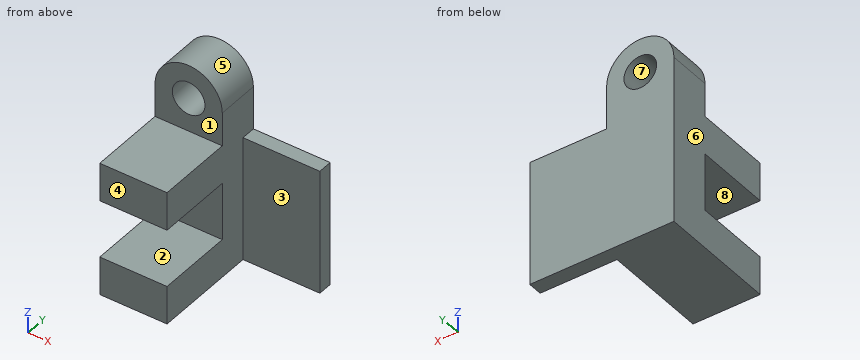
Autodesk Inventor part; units mm, degrees
ref_plane "YZ Plane" through (0, 0, 0) normal (1, 0, 0) x (0, 1, 0)
ref_plane "XZ Plane" through (0, 0, 0) normal (0, 1, 0) x (-1, 0, 0)
ref_plane "XY Plane" through (0, 0, 0) normal (0, 0, 1) x (1, 0, 0)
sketch "Sketch1" plane through (0, 0, 0) normal (0, 1, 0) x (-1, 0, 0)
  line L0 (0, -6.5) -> (-15, -6.5)
  line L1 (-15, -6.5) -> (-15, 6.5)
  line L2 (-15, 6.5) -> (0, 6.5)
  line L3 (0, 6.5) -> (0, -6.5)
  line L4 (0, -6.5) -> (-15, 6.5) construction
  line L5 (-15, -6.5) -> (0, 6.5) construction
  line L6 (0, -20.3) -> (0, 20.3)
  line L7 (-3.5, -11) -> (-3.5, 11) construction
  line L8 (0, -11) -> (0, -6.5) construction
  line L9 (-7, 11) -> (-7, -6.5)
  arc A0 (-7, -11) -> (0, -11) centre (-3.5, -11) ccw construction
  arc A1 (0, 11) -> (-7, 11) centre (-3.5, 11) ccw
  line L10 (0, -6.5) -> (0, 11)
  line L11 (-7, -6.5) -> (-7, -11) construction
  point P0 (0, 0)
  point P1 (-7.5, 0)
  point P2 (-7.5, 0)
  point P3 (-3.5, 0)
  point P4 (0, 11)
  point P5 (-7, 6.5)
  point P6 (0, 6.5)
  dimension "d0" = 13
  dimension "d1" = 15
  dimension "d3" = 7
  dimension "d4" = 8
  dimension "d5" = 8
extrude "Extrusion1" add sketch "Sketch1" along normal blind 1.5
sketch "Sketch2" plane through (0, 0, 0) normal (0, -1, 0) x (1, 0, 0)
  line L0 (7, 11) -> (7, 6.5)
  arc A0 (7, 11) -> (0, 11) centre (3.5, 11) ccw
  line L1 (0, -6.5) -> (0, 11)
  line L2 (15, -6.5) -> (0, -6.5)
  line L3 (15, 6.5) -> (15, -6.5)
  line L4 (7, 6.5) -> (15, 6.5)
  line L5 (7, 11) -> (7, 6.5)
  line L6 (7, 6.5) -> (7, -6.5)
  point P0 (0, 0)
extrude "Extrusion2" add sketch "Sketch2" along normal blind 3 contours L0 L6 L2 L1 A0
sketch "Sketch3" plane through (0, 1.5, -6.5) normal (-1, 0, 0) x (0, 0, 1)
  line L0 (14, -12.5) -> (10, -12.5)
  line L1 (10, -12.5) -> (10, -4.5)
  line L2 (10, -4.5) -> (14, -4.5)
  line L3 (14, -4.5) -> (14, -12.5)
  line L4 (17.5, -4.5) -> (0, -4.5)
  line L5 (13, -1.5) -> (13, 0)
  line L6 (0, -4.5) -> (4, -4.5)
  line L7 (4, -4.5) -> (4, -12.5)
  line L8 (4, -12.5) -> (0, -12.5)
  line L9 (0, -12.5) -> (0, -4.5)
  point P0 (6.5, -1.5)
  dimension "d10" = 4
  dimension "d11" = 8
  dimension "d12" = 1
  dimension "d13" = 4
extrude "Extrusion3" add sketch "Sketch3" against normal up to surface (7 mm away)
sketch "Sketch4" plane through (0, -3, 0) normal (0, -1, 0) x (1, 0, 0)
  arc A0 (7, 11) -> (0, 11) centre (3.5, 11) ccw
  point P0 (0, 0)
hole "Hole1" at (3.5, -3, 11) direction (0, 1, 0) diameter 3.4 end through all
equation "\"d5\" = d4"
equation "\"d13\" = d10"
properties part number "optical sensor"
Design review of the part built by this model. Coordinates are the model's own, in mm. Face numbers are marked on the shaded views. A direction names the side the tool comes from. Give positions to 0.01 mm unless a question says otherwise; leave off trailing zeros. Loops run counter-clockwise (first coordinate to the right, second up) from the corner with the lowest first, then second, coordinate; pieces in that order, holes last. Notation, with made-up numbers: M 61.5,-18 L 116.5,-18 A33 ccw 116.5,15 Z; hole C 6.5,-12.75 d11. An arc over 180 degrees is marked long. Return JSON: item names as keys, results as strings. Group by question number.
Item 1: Mouldability with a two-part tool opening along X and no side actions: class the marked faces 5, 6, 7 and 8 as released by +X, released by -X, zero draft, split by the parting line, or undercut.
Item 2: We need section B-B (x = 3.5). Give the boundary of the cut face in (y, z), and give its area (3 significant figures).
Item 3: We need section C-C (z = 11.5). Give the boundary of the cut face in (x, y).
Item 4: For probe 1 along Z at (x, y) = (3.5, -1.2); probe 2 along X at (y, z) = (-0.5, 11); probe 3 along Z at (x, y) = (1.75, -6.5), list the stretches that pass through material, from the lowest coordinate up.
Item 5: Tool access review of the marked faces 1, 2, 3 and 4: name each direction out of +Z, -Z, +X, -X, +Y, -Y from which nothing blocks a thin tool from reaching the whole face with its end or side.
Item 6: We need section D-D (y = -1.5). Give the boundary of the cut face in (x, z).
Item 7: Insertion check: pin 1 Ø1.5 at (x, z) = (10, 4) entering from -Y; pin 2 Ø7.5 at (x, y) = (3.5, -8.5) entering from +Z; pin 3 Ø3.5 at (x, z) = (3, 11.5) entering from -Y. Each pin has a flat end and moves straight along its axis. Give the tip position at first contact, or say it passes through.
Item 8: We need section A-A (y = -6.25). Give the boundary of the cut face in (x, z).
Output:
{
 "1": {"face 5": "split by the parting line", "face 6": "released by -X", "face 7": "undercut", "face 8": "zero draft"},
 "2": {"outline": "M -11,-6.5 L 1.5,-6.5 L 1.5,9.3 L -3,9.3 L -3,7.5 L -11,7.5 L -11,3.5 L -3,3.5 L -3,-2.5 L -11,-2.5 Z; M -3,12.7 L 1.5,12.7 L 1.5,14.5 L -3,14.5 Z", "area": "143 mm^2"},
 "3": {"outline": "M 0.04,-3 L 1.88,-3 L 1.88,1.5 L 0.04,1.5 Z; M 5.12,-3 L 6.96,-3 L 6.96,1.5 L 5.12,1.5 Z"},
 "4": {"probe 1": "z = -6.5 to 9.3, 12.7 to 14.5", "probe 2": "x = 0 to 1.8, 5.2 to 7", "probe 3": "z = -6.5 to -2.5, 3.5 to 7.5"},
 "5": {"face 1": "+Z, +X, -X, -Y", "face 2": "+X, -X, -Y", "face 3": "+Z, -Z, +X, -Y", "face 4": "+Z, -Z, +X, -X, -Y"},
 "6": {"outline": "M 0,-6.5 L 7,-6.5 L 7,11 A3.5 ccw 0,11 Z; hole C 3.5,11 d3.4"},
 "7": {"pin 1": "stops at y = 0", "pin 2": "stops at z = 7.5", "pin 3": "stops at y = -3"},
 "8": {"outline": "M 0,-6.5 L 7,-6.5 L 7,-2.5 L 0,-2.5 Z; M 0,3.5 L 7,3.5 L 7,7.5 L 0,7.5 Z"}
}
